Read the model definition and answer for the solid it produces. Units are mm, in the model's axes. Round coordinates to 2 decimals unless told otherwise and drop trailing zeros. Order: outer loops, then holes, each group sorted by start corner. A loop starts at its lowest first (then second) coordinate and runs counter-clockwise, first axis right, second up. Notation, with made-up numbers: (81.5, -16.75) - (129.5, -16.75) arc R23 ccw to (129.5, -8.75) - close; hole circle Ø8 at (-12.5, 8.5). An arc over 180 degrees is marked (long way). Answer as a JSON object with one key per item and string values. Group by question number.
Q1. A cutting plane is placed at B-B on z = 38.1. Determine the outline of the cut face in (x, y) (3 decimals).
Q2. A cutting plane is placed at A-A on x = -190.5. Determine the outline of the cut face in (y, z) (3 decimals), and give its area (3 significant figures).
Q3. A cutting plane is placed at C-C on y = 1. Count the separate pieces of the cut face and the enclosed holes in it, and give its area (3 significant figures).
Q4. Given pin 1 Ø10.5 at (x, z) = (-266.7, -190.5) entering from -Y; pin 2 Ø1 at (y, z) = (0, -130) entering from +X, each flat-ended and moving along its own axis, determine where each tip first touches the part or whether it passes through.
Q5. Consider line 1 (X direction, y = -1.5, z = 184.15); line 2 (X direction, y = -1, z = 0); line 3 (Z direction, x = 138, y = 2.25). Determine where each line is inside the solid, lowest interval first.
Q6. A cutting plane is placed at D-D on z = -62. Determine the outline of the cut face in (x, y) (3 decimals).
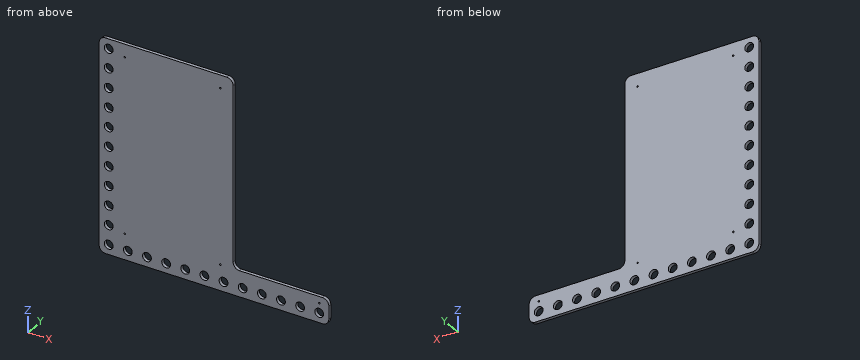
```python
from build123d import *

# Parameters (mm, degrees)
SKETCH1_W           = 571.5
SKETCH1_H           = 419.1
BOSS_EXTRUDE1_DEPTH = 3.175
SKETCH2_R           = 4.4196
CUT_EXTRUDE1_DEPTH  = 355.407375064
SKETCH3_R           = 8.73125
CUT_EXTRUDE2_DEPTH  = 355.407375064
CUT_EXTRUDE5_DEPTH  = 355.407375064
SKETCH5_R           = 1.5113
CUT_EXTRUDE3_DEPTH  = 355.407375064
FILLET1_R           = 12.7


with BuildPart() as part:
    # Sketch1 → Boss-Extrude1 (new, symmetric)
    with BuildSketch(Plane(origin=(0, 0, 0), x_dir=(1, 0, 0), z_dir=(0, 1, 0))):
        Rectangle(SKETCH1_W, SKETCH1_H)
    extrude(amount=BOSS_EXTRUDE1_DEPTH, both=True)

    # Sketch2 → Cut-Extrude1 (cut, through all)
    with BuildSketch(Plane(origin=(0, 3.175, 0), x_dir=(1, 0, 0), z_dir=(0, 1, 0))):
        with Locations(Location((-228.6, 190.5, 0), (0, 0, 270))):
            Circle(SKETCH2_R)
        with Locations(Location((-190.5, 190.5, 0), (0, 0, 270))):
            Circle(SKETCH2_R)
        with Locations(Location((-152.4, 190.5, 0), (0, 0, 270))):
            Circle(SKETCH2_R)
        with Locations(Location((-114.3, 190.5, 0), (0, 0, 270))):
            Circle(SKETCH2_R)
        with Locations(Location((-76.2, 190.5, 0), (0, 0, 270))):
            Circle(SKETCH2_R)
        with Locations(Location((-38.1, 190.5, 0), (0, 0, 270))):
            Circle(SKETCH2_R)
        with Locations(Location((0, 190.5, 0), (0, 0, 270))):
            Circle(SKETCH2_R)
        with Locations(Location((38.1, 190.5, 0), (0, 0, 270))):
            Circle(SKETCH2_R)
        with Locations(Location((-266.7, 38.1, 0), (0, 0, 270))):
            Circle(SKETCH2_R)
        with Locations(Location((-266.7, 76.2, 0), (0, 0, 270))):
            Circle(SKETCH2_R)
        with Locations(Location((-266.7, 114.3, 0), (0, 0, 270))):
            Circle(SKETCH2_R)
        with Locations(Location((-266.7, 152.4, 0), (0, 0, 270))):
            Circle(SKETCH2_R)
        with Locations(Location((-266.7, 190.5, 0), (0, 0, 270))):
            Circle(SKETCH2_R)
        with Locations(Location((-266.7, -190.5, 0), (0, 0, 90))):
            Circle(SKETCH2_R)
        with Locations(Location((-266.7, -152.4, 0), (0, 0, 90))):
            Circle(SKETCH2_R)
        with Locations(Location((-266.7, -114.3, 0), (0, 0, 90))):
            Circle(SKETCH2_R)
        with Locations(Location((-266.7, -76.2, 0), (0, 0, 90))):
            Circle(SKETCH2_R)
        with Locations(Location((-266.7, -38.1, 0), (0, 0, 90))):
            Circle(SKETCH2_R)
        with Locations(Location((-266.7, 0, 0), (0, 0, 90))):
            Circle(SKETCH2_R)
        with Locations(Location((76.2, 190.5, 0), (0, 0, 270))):
            Circle(SKETCH2_R)
        with Locations(Location((114.3, 190.5, 0), (0, 0, 270))):
            Circle(SKETCH2_R)
        with Locations(Location((152.4, 190.5, 0), (0, 0, 270))):
            Circle(SKETCH2_R)
        with Locations(Location((190.5, 190.5, 0), (0, 0, 270))):
            Circle(SKETCH2_R)
        with Locations(Location((228.6, 190.5, 0), (0, 0, 270))):
            Circle(SKETCH2_R)
        with Locations(Location((266.7, 190.5, 0), (0, 0, 270))):
            Circle(SKETCH2_R)
    extrude(amount=-CUT_EXTRUDE1_DEPTH, mode=Mode.SUBTRACT)

    # Sketch3 → Cut-Extrude2 (cut, through all)
    with BuildSketch(Plane(origin=(0, 3.175, 0), x_dir=(1, 0, 0), z_dir=(0, 1, 0))):
        with Locations(Location((-266.7, 190.5, 0), (0, 0, 270))):
            Circle(SKETCH3_R)
        with Locations(Location((-228.6, 190.5, 0), (0, 0, 270))):
            Circle(SKETCH3_R)
        with Locations(Location((-190.5, 190.5, 0), (0, 0, 270))):
            Circle(SKETCH3_R)
        with Locations(Location((-152.4, 190.5, 0), (0, 0, 270))):
            Circle(SKETCH3_R)
        with Locations(Location((-114.3, 190.5, 0), (0, 0, 270))):
            Circle(SKETCH3_R)
        with Locations(Location((-76.2, 190.5, 0), (0, 0, 270))):
            Circle(SKETCH3_R)
        with Locations(Location((-38.1, 190.5, 0), (0, 0, 270))):
            Circle(SKETCH3_R)
        with Locations(Location((0, 190.5, 0), (0, 0, 270))):
            Circle(SKETCH3_R)
        with Locations(Location((38.1, 190.5, 0), (0, 0, 270))):
            Circle(SKETCH3_R)
        with Locations(Location((76.2, 190.5, 0), (0, 0, 270))):
            Circle(SKETCH3_R)
        with Locations(Location((114.3, 190.5, 0), (0, 0, 270))):
            Circle(SKETCH3_R)
        with Locations(Location((152.4, 190.5, 0), (0, 0, 270))):
            Circle(SKETCH3_R)
        with Locations(Location((190.5, 190.5, 0), (0, 0, 270))):
            Circle(SKETCH3_R)
        with Locations(Location((228.6, 190.5, 0), (0, 0, 270))):
            Circle(SKETCH3_R)
        with Locations(Location((266.7, 190.5, 0), (0, 0, 270))):
            Circle(SKETCH3_R)
        with Locations(Location((-266.7, 152.4, 0), (0, 0, 270))):
            Circle(SKETCH3_R)
        with Locations(Location((-266.7, 114.3, 0), (0, 0, 270))):
            Circle(SKETCH3_R)
        with Locations(Location((-266.7, 76.2, 0), (0, 0, 270))):
            Circle(SKETCH3_R)
        with Locations(Location((-266.7, 38.1, 0), (0, 0, 270))):
            Circle(SKETCH3_R)
        with Locations(Location((-266.7, 0, 0), (0, 0, 270))):
            Circle(SKETCH3_R)
        with Locations(Location((-266.7, -38.1, 0), (0, 0, 270))):
            Circle(SKETCH3_R)
        with Locations(Location((-266.7, -76.2, 0), (0, 0, 270))):
            Circle(SKETCH3_R)
        with Locations(Location((-266.7, -114.3, 0), (0, 0, 270))):
            Circle(SKETCH3_R)
        with Locations(Location((-266.7, -152.4, 0), (0, 0, 270))):
            Circle(SKETCH3_R)
        with Locations(Location((-266.7, -190.5, 0), (0, 0, 270))):
            Circle(SKETCH3_R)
    extrude(amount=-CUT_EXTRUDE2_DEPTH, mode=Mode.SUBTRACT)

    # Sketch8 → Cut-Extrude5 (cut, through all)
    with BuildSketch(Plane(origin=(0, 3.175, 0), x_dir=(1, 0, 0), z_dir=(0, 1, 0))):
        Polygon((-19.05, -209.55), (285.75, -209.55), (285.75, 209.55), (171.45, 209.55), (171.45, 158.75), (-19.05, 158.75), align=None)
    extrude(amount=-CUT_EXTRUDE5_DEPTH, mode=Mode.SUBTRACT)

    # Sketch5 → Cut-Extrude3 (cut, through all)
    with BuildSketch(Plane(origin=(0, 3.175, 0), x_dir=(1, 0, 0), z_dir=(0, 1, 0))):
        with Locations(Location((-234.95, -184.15, 0), (0, 0, 270))):
            Circle(SKETCH5_R)
        with Locations(Location((-234.95, 158.75, 0), (0, 0, 270))):
            Circle(SKETCH5_R)
        with Locations(Location((-44.45, -184.15, 0), (0, 0, 270))):
            Circle(SKETCH5_R)
        with Locations(Location((-44.45, 158.75, 0), (0, 0, 270))):
            Circle(SKETCH5_R)
        with Locations(Location((152.4, 171.45, 0), (0, 0, 270))):
            Circle(SKETCH5_R)
    extrude(amount=-CUT_EXTRUDE3_DEPTH, mode=Mode.SUBTRACT)

    # Fillet1
    fillet1_edges = [part.edges().sort_by_distance(p)[0] for p in [
        (-19.05, 0, 209.55),
        (-19.05, 0, -158.75),
        (171.45, 0, -158.75),
        (171.45, 0, -209.55),
        (-285.75, 0, 209.55),
        (-285.75, 0, -209.55),
    ]]
    fillet(fillet1_edges, radius=FILLET1_R)


solid = part.part
```
Result set:
{
 "1": {"outline": "(-285.75, -3.175) - (-275.431, -3.175) - (-275.431, 3.175) - (-285.75, 3.175) - close; (-257.969, -3.175) - (-19.05, -3.175) - (-19.05, 3.175) - (-257.969, 3.175) - close"},
 "2": {"outline": "(-3.175, -209.55) - (3.175, -209.55) - (3.175, -199.231) - (-3.175, -199.231) - close; (-3.175, -181.769) - (3.175, -181.769) - (3.175, 209.55) - (-3.175, 209.55) - close", "area": "2,550 mm²"},
 "3": {"separate pieces": "1", "enclosed holes": "27", "area": "116,000 mm²"},
 "4": {"pin 1": "passes through", "pin 2": "stops at x = -19.05"},
 "5": {"line 1": "x = -285.75 to -272.69, -260.71 to -236.46, -233.44 to -45.96, -42.94 to -19.05", "line 2": "x = -285.75 to -275.43, -257.97 to -19.05", "line 3": "z = -209.55 to -158.75"},
 "6": {"outline": "(-285.75, -3.175) - (-19.05, -3.175) - (-19.05, 3.175) - (-285.75, 3.175) - close"}
}
